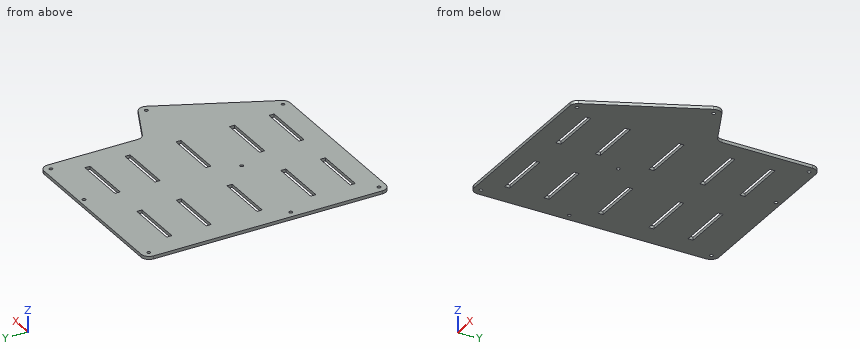
```python
from build123d import *

# Parameters (mm, degrees)
SKETCH1_R           = 1.5
SKETCH1_W           = 45.562449769
SKETCH1_H           = 4.5
BOSS_EXTRUDE1_DEPTH = 2.7


with BuildPart() as part:
    # Sketch1 → Boss-Extrude1 (new body)
    with BuildSketch(Plane.XY):
        with BuildLine():
            Line((181.0868, 176.698), (181.0868, 97.809302293))
            ThreePointArc((181.0868, 97.809302293), (182.183121351, 94.048108544), (185.128679547, 91.465051085))
            Line((185.128679547, 91.465051085), (218.538914615, 75.886932175))
            ThreePointArc((218.538914615, 75.886932175), (222.158599458, 71.936940245), (221.924958355, 66.584373903))
            Line((221.924958355, 66.584373903), (178.566520277, -26.398891285))
            ThreePointArc((178.566520277, -26.398891285), (175.983463005, -29.344318185), (172.222356084, -30.44058422))
            Line((172.222356084, -30.44058422), (27, -30.44058422))
            ThreePointArc((27, -30.44058422), (22.050252532, -28.390331688), (20, -23.44058422))
            Line((20, -23.44058422), (20, 176.698))
            ThreePointArc((20, 176.698), (22.050252532, 181.647747468), (27, 183.698))
            Line((27, 183.698), (174.0868, 183.698))
            ThreePointArc((174.0868, 183.698), (179.036547468, 181.647747468), (181.0868, 176.698))
        make_face()
        with Locations(Location((216.558534729, 69.898485122, 0), (0, 0, 180))):
            Circle(SKETCH1_R, mode=Mode.SUBTRACT)
        with Locations(Location((106.66988, 49.713, 0), (0, 0, 180))):
            Circle(SKETCH1_R, mode=Mode.SUBTRACT)
        with Locations(Location((26.263876, 53.119376266, 0), (0, 0, 180))):
            Circle(SKETCH1_R, mode=Mode.SUBTRACT)
        with Locations(Location((26.263876266, 177.434123734, 0), (0, 0, 180))):
            Circle(SKETCH1_R, mode=Mode.SUBTRACT)
        with Locations(Location((121.3333, 179.253, 0), (0, 0, 180))):
            Circle(SKETCH1_R, mode=Mode.SUBTRACT)
        with Locations(Location((174.816573734, 177.434123734, 0), (0, 0, 180))):
            Circle(SKETCH1_R, mode=Mode.SUBTRACT)
        with Locations(Location((26.263876, -24.17668422, 0), (0, 0, 180))):
            Circle(SKETCH1_R, mode=Mode.SUBTRACT)
        with Locations(Location((172.941013343, -24.56864608, 0), (0, 0, 180))):
            Circle(SKETCH1_R, mode=Mode.SUBTRACT)
        with Locations((140.588022236, 151.948)):
            Rectangle(SKETCH1_W, SKETCH1_H, mode=Mode.SUBTRACT)
        with Locations((62.781224885, 151.448)):
            Rectangle(SKETCH1_W, SKETCH1_H, mode=Mode.SUBTRACT)
        with Locations((62.781224885, 116.948)):
            Rectangle(SKETCH1_W, SKETCH1_H, mode=Mode.SUBTRACT)
        with Locations((62.781224885, 72.448)):
            Rectangle(SKETCH1_W, SKETCH1_H, mode=Mode.SUBTRACT)
        with Locations((62.781224885, 25.448)):
            Rectangle(SKETCH1_W, SKETCH1_H, mode=Mode.SUBTRACT)
        with Locations((62.781224885, -9.052)):
            Rectangle(SKETCH1_W, SKETCH1_H, mode=Mode.SUBTRACT)
        with Locations((140.588022236, 116.948)):
            Rectangle(SKETCH1_W, SKETCH1_H, mode=Mode.SUBTRACT)
        with Locations((140.588022236, 72.448)):
            Rectangle(SKETCH1_W, SKETCH1_H, mode=Mode.SUBTRACT)
        with Locations((140.588022236, 25.448)):
            Rectangle(SKETCH1_W, SKETCH1_H, mode=Mode.SUBTRACT)
        with Locations((140.588022236, -9.052)):
            Rectangle(SKETCH1_W, SKETCH1_H, mode=Mode.SUBTRACT)
    extrude(amount=BOSS_EXTRUDE1_DEPTH)


solid = part.part
```
Here's how the part is built. I have some questions about the finished solid (model axes, mm). Give positions to 0.01 mm unless a question says otherwise; leave off trailing zeros. Loops run counter-clockwise (first coordinate to the right, second up) from the corner with the lowest first, then second, coordinate; pieces in that order, holes last. Notation, with made-up numbers: M 69,35.25 L 125,35.25 A35 cw 125,69.25 Z; hole C -24,14 d8. An arc over 180 degrees is marked long. Use one line per item in the form item = value. Start each with the question number.
Q1. I need wall thicknesses on line 1 along Y through (x, z) = (119.5, 1.7); line 2 along Y through (x, z) = (44.5, 1.7); line 3 along X through (y, z) = (151, 2.6). Which ranges of each line are inside material? Lowest first, please.
Q2. If we section it at C-C (z = 1): State how many separate pieces and enclosed holes the cut face has, then the cut area to 3 significant figures.
Q3. If we section it at D-D (x = 209): Write out the boundary of the cut face in (y, z), then the cut area to 3 significant figures.
Q4. If we section it at A-A (x = 70): Write out the boundary of the cut face in (y, z).
Q5. Will these pins go through, and if not, where does the flat tip stop? pin 1 Ø1.4 at (y, z) = (118, 1.5) entering from +X; pin 2 Ø1.4 at (y, z) = (73, 1) entering from +X.
Q6. If we section it at B-B (y = 137): Write out the boundary of the cut face in (x, z).
Taken from the geometry:
q1.line_1 = -30.44 to -11.3, -6.8 to 23.2, 27.7 to 70.2, 74.7 to 114.7, 119.2 to 149.7, 154.2 to 183.7
q1.line_2 = -30.44 to -11.3, -6.8 to 23.2, 27.7 to 70.2, 74.7 to 114.7, 119.2 to 149.2, 153.7 to 183.7
q1.line_3 = 20 to 40, 85.56 to 117.81, 163.37 to 181.09
q2.separate_pieces = 1
q2.enclosed_holes = 18
q2.area = 34,800 mm^2
q3.outline = M 38.87,0 L 80.33,0 L 80.33,2.7 L 38.87,2.7 Z
q3.area = 112 mm^2
q4.outline = M -30.44,0 L -11.3,0 L -11.3,2.7 L -30.44,2.7 Z; M -6.8,0 L 23.2,0 L 23.2,2.7 L -6.8,2.7 Z; M 27.7,0 L 70.2,0 L 70.2,2.7 L 27.7,2.7 Z; M 74.7,0 L 114.7,0 L 114.7,2.7 L 74.7,2.7 Z; M 119.2,0 L 149.2,0 L 149.2,2.7 L 119.2,2.7 Z; M 153.7,0 L 183.7,0 L 183.7,2.7 L 153.7,2.7 Z
q5.pin_1 = 181.09
q5.pin_2 = 222.01
q6.outline = M 20,0 L 181.09,0 L 181.09,2.7 L 20,2.7 Z
